```python
from build123d import *

# Parameters (mm, degrees)
SKETCH1_W           = 12
SKETCH1_H           = 6
BOSS_EXTRUDE1_DEPTH = 30
SKETCH2_W           = 12
SKETCH2_H           = 10
BOSS_EXTRUDE2_DEPTH = 5
CUT_EXTRUDE1_DEPTH  = 34.286633954
FILLET1_R           = 5


with BuildPart() as part:
    # Sketch1 → Boss-Extrude1 (new body)
    with BuildSketch(Plane.XY):
        Rectangle(SKETCH1_W, SKETCH1_H)
    extrude(amount=-BOSS_EXTRUDE1_DEPTH)

    # Sketch2 → Boss-Extrude2 (add)
    with BuildSketch(Plane(origin=(0, 3, 0), x_dir=(1, 0, 0), z_dir=(0, 1, 0))):
        with Locations((0, 5)):
            Rectangle(SKETCH2_W, SKETCH2_H)
    extrude(amount=BOSS_EXTRUDE2_DEPTH)

    # Sketch3 → Cut-Extrude1 (cut, through all)
    with BuildSketch(Plane(origin=(6, 0, 0), x_dir=(0, 0, -1), z_dir=(1, 0, 0))):
        Polygon((5, 8), (0, 3), (0, 8), align=None)
    extrude(amount=-CUT_EXTRUDE1_DEPTH, mode=Mode.SUBTRACT)

    # Fillet1
    fillet1_edges = [part.edges().sort_by_distance(p)[0] for p in [
        (-6, 0, -30),
        (6, 0, -30),
    ]]
    fillet(fillet1_edges, radius=FILLET1_R)


solid = part.part
```
Source: CAD feature listing. Evaluate the final solid. Frame: model axes, mm. A direction names the side the tool comes from. Coordinates: 2 decimals unless noted, no trailing zeros. Write each loop counter-clockwise with the first axis right and the second up, starting at its lowest first coordinate (ties: lowest second). Pieces come first, ordered by that corner, then holes. Notation, with made-up numbers: (40, 10.5) - (97, 10.5) arc R22 ccw to (97, 37.5) - close; hole circle Ø7 at (81, -14). An arc over 180 degrees is marked (long way). Answer as a JSON object with one key per item and string values.
Q1. First-contact query: pin 1 Ø2.5 at (x, y) = (-1.5, 6.5) entering from -Z. Flat tip, straight axial feed; report the tip coordinate or a pass-through.
Ans:
{"pin 1": "stops at z = -10"}
Q2. Material intervals for line 1 (Y direction, x = -5.5, z = -14.25); line 2 (Z direction, x = -3.25, y = 4); line 3 (Z direction, x = 0, y = 6), sorted ascending. Write a range as [from, to].
Ans:
{"line 1": "y = [-3, 3]", "line 2": "z = [-10, -1]", "line 3": "z = [-10, -3]"}
Q3. Section query D-D, the plane x = -4. Output: boundary loops of the cut face in (y, z).
Ans:
{"outline": "(-3, -29) - (3, -29) - (3, -10) - (8, -10) - (8, -5) - (3, 0) - (-3, 0) - close"}
Q4. Section query B-B, the plane y = 2. Output: boundary loops of the cut face in (x, z).
Ans:
{"outline": "(-6, -25) arc R5 ccw to (-1, -30) - (1, -30) arc R5 ccw to (6, -25) - (6, 0) - (-6, 0) - close"}
Q5. Set-up query: faces 1 (the flat face through (0, 3, -20)), 2 (the flat face through (0, 0, -30)). Return all of +Z, -Z, +X, -X, +Y, -Y with unobstructed straight access to the full face (end or side cutting, diameter ignored); none if empty.
Ans:
{"face 1": "-Z, +X, -X, +Y", "face 2": "-Z, +X, -X, +Y, -Y"}
Q6. Section query A-A, the plane x = 0. Output: boundary loops of the cut face in (y, z).
Ans:
{"outline": "(-3, -30) - (3, -30) - (3, -10) - (8, -10) - (8, -5) - (3, 0) - (-3, 0) - close"}
Q7. Section query C-C, the plane z = -12.5. Output: boundary loops of the cut face in (x, y).
Ans:
{"outline": "(-6, -3) - (6, -3) - (6, 3) - (-6, 3) - close"}
